```python
from build123d import *

# Parameters (mm, degrees)
SKETCH2_W                = 75
SKETCH2_H                = 75
SKETCH2_R                = 21
BOSS_EXTRUDE1_DEPTH      = 6
M4_CLEARANCE_HOLE1_D     = 4.8
M4_CLEARANCE_HOLE1_DEPTH = 25
FILLET1_R                = 6.35
SKETCH5_R                = 22.809118079
BOSS_EXTRUDE2_DEPTH      = 19
FILLET2_R                = 10
M5_TAPPED_HOLE1_D        = 4.2
M5_TAPPED_HOLE1_DEPTH    = 12.4
M5_TAPPED_HOLE1_TIP      = 1.2618073


with BuildPart() as part:
    # Sketch1 → Revolve1 (revolve)
    with BuildSketch(Plane.XY, mode=Mode.PRIVATE) as revolve1_sk:
        Polygon((-16.5, 0), (-34, 0), (-34, 6), (-24, 6), (-24, 25), (-18.5, 25), (-18.5, 13), (-16.5, 13), align=None)
    revolve(revolve1_sk.sketch.rotate(Axis((0, 0, 0), (0, 1, 0)), 270), axis=Axis((0, 0, 0), (0, 1, 0)))

    # Sketch2 → Boss-Extrude1 (add)
    with BuildSketch(Plane(origin=(0, 6, 0), x_dir=(1, 0, 0), z_dir=(0, 1, 0))):
        Rectangle(SKETCH2_W, SKETCH2_H)
        Circle(SKETCH2_R, mode=Mode.SUBTRACT)
    extrude(amount=-BOSS_EXTRUDE1_DEPTH)

    # M4 Clearance Hole1
    with Locations(Plane(origin=(0, 0, 0), x_dir=(-1, 0, 0), z_dir=(0, -1, 0))):
        with Locations((0, 0), (-31.819805153, 31.819805153), (31.819805153, 31.819805153), (31.819805153, -31.819805153), (-31.819805153, -31.819805153)):
            Hole(M4_CLEARANCE_HOLE1_D / 2, depth=M4_CLEARANCE_HOLE1_DEPTH)

    # Fillet1
    fillet1_edges = [part.edges().sort_by_distance(p)[0] for p in [
        (37.5, 3, 37.5),
        (37.5, 3, -37.5),
        (-37.5, 3, -37.5),
        (-37.5, 3, 37.5),
    ]]
    fillet(fillet1_edges, radius=FILLET1_R)

    # Sketch5 → Boss-Extrude2 (add)
    with BuildSketch(Plane(origin=(0, 25, 0), x_dir=(1, 0, 0), z_dir=(0, 1, 0))):
        with BuildLine():
            Line((0, 24), (6.5, 24))
            Line((6.5, 24), (30.5, 24))
            Line((30.5, 24), (30.5, -24))
            Line((30.5, -24), (6.5, -24))
            Line((6.5, -24), (0, -24))
            ThreePointArc((0, -24), (-24, 0), (0, 24))
        make_face()
        Circle(SKETCH5_R, mode=Mode.SUBTRACT)
    extrude(amount=-BOSS_EXTRUDE2_DEPTH)

    # Fillet2
    fillet2_edges = [part.edges().sort_by_distance(p)[0] for p in [
        (30.5, 15.5, -24),
        (30.5, 15.5, 24),
    ]]
    fillet(fillet2_edges, radius=FILLET2_R)

    # M5 Tapped Hole1
    with Locations(Plane(origin=(0, 25, 0), x_dir=(1, 0, 0), z_dir=(0, 1, 0))):
        with Locations((22.5, 16), (22.5, -16)):
            Hole(M5_TAPPED_HOLE1_D / 2, depth=M5_TAPPED_HOLE1_DEPTH)
            with Locations((0, 0, -(M5_TAPPED_HOLE1_DEPTH + M5_TAPPED_HOLE1_TIP / 2))):  # 118° drill point
                Cone(0, M5_TAPPED_HOLE1_D / 2, M5_TAPPED_HOLE1_TIP, mode=Mode.SUBTRACT)


solid = part.part
```
Input: part model. Units: mm. Frame: model coordinates. A direction names the side the tool comes from. Round coordinates to 2 decimals unless told otherwise and drop trailing zeros. Loops run counter-clockwise (first coordinate to the right, second up) from the corner with the lowest first, then second, coordinate; pieces in that order, holes last. Notation, with made-up numbers: (-33, 78) -> (-9, 78) arc R29 ccw to (-9, 103) -> close; hole circle Ø11 at (-30, 25.25). An arc over 180 degrees is marked (long way). Use one line per item in the form item = value. Start each with the question number.
Item 1: Section query A-A on z = 0. Return the cut outline in (x, y), then the cut area to 4 significant figures.
Item 2: Section query B-B on y = 19.5. Return the cut outline in (x, z).
Item 3: Material intervals for L1, parallel to Z at x = 21.5, y = 21; L2, parallel to X at y = 19.75, z = -16; L3, parallel to Z at x = 22.5, y = 22.25, sorted ascending. Write a range as from..to.
Item 4: Section query D-D on y = 4.75. Return the cut outline in (x, z).
Item 5: Section query C-C on x = -3. Return the cut outline in (y, z), then the cut area to 3 significant figures.
Item 6: Contact query for flat-ended pins moving along their axis: pin 1 Ø4.5 at (x, z) = (31.82, -31.82) entering from -Y; pin 2 Ø1.5 at (x, z) = (-13.5, 30) entering from +Y; pin 3 Ø5.5 at (x, y) = (12, 17) entering from -Z; pin 4 Ø1 at (y, z) = (19, 9) entering from +X. Output: stop coordinate, or through.
Item 7: Set-up query: faces 1 (the face through (-23.994, 15.633, -0.528)), 2 (the face through (27.65, 15.37, 20.99)), 3 (the face through (21.37, 18.71, -17.77)), 4 (the face through (27.49, 15.37, -21.15)). Return all of +Z, -Z, +X, -X, +Y, -Y with unobstructed straight access to the full face (end or side cutting, diameter ignored); none if empty.
Item 8: Mould query, pull axis Z, two halves, no side actions, for faces 5 (the face through (22.773, 18.713, 13.918)), 6 (the face through (-35.69, 2.96, -35.59)), 7 (the face through (16.108, 6.409, 3.577)), 8 (the face through (30.5, 16, 0)). Classes: pulls with the +Z half, pulls with the -Z half, needs draft (parallel to the pull), parting line crosses it, or undercut.
Ans:
q1.outline = (-37.5, 0) -> (-16.5, 0) -> (-16.5, 13) -> (-18.5, 13) -> (-18.5, 25) -> (-24, 25) -> (-24, 6) -> (-37.5, 6) -> close; (16.5, 0) -> (37.5, 0) -> (37.5, 6) -> (30.5, 6) -> (30.5, 25) -> (18.5, 25) -> (18.5, 13) -> (16.5, 13) -> close
q1.area = 612.5 mm^2
q2.outline = (0, -24) -> (20.5, -24) arc R10 ccw to (30.5, -14) -> (30.5, 14) arc R10 ccw to (20.5, 24) -> (0, 24) arc R24 ccw to start; hole circle Ø37 at (0, 0); hole circle Ø4.2 at (22.5, -16); hole circle Ø4.2 at (22.5, 16)
q3.L1 = -23.95..-17.85, -14.15..14.15, 17.85..23.95
q3.L2 = -17.89..-9.29, 9.29..20.4, 24.6..30.3
q3.L3 = -23.8..-18.1, -13.9..13.9, 18.1..23.8
q4.outline = (-37.5, -31.15) arc R6.35 ccw to (-31.15, -37.5) -> (31.15, -37.5) arc R6.35 ccw to (37.5, -31.15) -> (37.5, 31.15) arc R6.35 ccw to (31.15, 37.5) -> (-31.15, 37.5) arc R6.35 ccw to (-37.5, 31.15) -> close; hole circle Ø4.8 at (-31.82, -31.82); hole circle Ø4.8 at (-31.82, 31.82); hole circle Ø33 at (0, 0); hole circle Ø4.8 at (31.82, -31.82); hole circle Ø4.8 at (31.82, 31.82)
q5.outline = (0, -37.5) -> (6, -37.5) -> (6, -23.81) -> (25, -23.81) -> (25, -18.26) -> (13, -18.26) -> (13, -16.22) -> (0, -16.22) -> close; (0, 16.22) -> (13, 16.22) -> (13, 18.26) -> (25, 18.26) -> (25, 23.81) -> (6, 23.81) -> (6, 37.5) -> (0, 37.5) -> close
q5.area = 495 mm^2
q6.pin_1 = through
q6.pin_2 = 6
q6.pin_3 = -24
q6.pin_4 = 30.5
q7.face_1 = -X, +Y
q7.face_2 = +Z, +X, +Y
q7.face_3 = +Y
q7.face_4 = -Z, +X, +Y
q8.face_5 = undercut
q8.face_6 = pulls with the -Z half
q8.face_7 = undercut
q8.face_8 = needs draft
